CAD build for the part. Positions are in the model's coordinates, mm. Coordinates: 2 decimals unless noted, no trailing zeros. Loops run counter-clockwise (first coordinate to the right, second up) from the corner with the lowest first, then second, coordinate; pieces in that order, holes last. Notation, with made-up numbers: M -32.75,62 L -3.75,62 A7 ccw -3.75,69 Z; hole C -15.5,-17.5 d8. An arc over 180 degrees is marked long. Answer as a JSON object with one key per item and string values. Group by question number.
Autodesk Inventor part; units mm, degrees
ref_plane "YZ Plane" through (0, 0, 0) normal (1, 0, 0) x (0, 1, 0)
ref_plane "XZ Plane" through (0, 0, 0) normal (0, 1, 0) x (-1, 0, 0)
ref_plane "XY Plane" through (0, 0, 0) normal (0, 0, 1) x (1, 0, 0)
sketch "Sketch1" plane through (0, 0, 0) normal (0, 1, 0) x (-1, 0, 0)
  line L0 (50, 50) -> (-50, 50)
  line L1 (-50, 50) -> (-50, -50)
  line L2 (-50, -50) -> (50, -50)
  line L3 (50, -50) -> (50, 50)
  line L4 (50, 50) -> (-50, -50) construction
  line L5 (-50, 50) -> (50, -50) construction
  line L6 (100, 100) -> (-100, 100)
  line L7 (-100, 100) -> (-100, -100)
  line L8 (-100, -100) -> (100, -100)
  line L9 (100, -100) -> (100, 100)
  line L10 (100, 100) -> (-100, -100) construction
  line L11 (-100, 100) -> (100, -100) construction
  line L12 (-50, 100) -> (-260, 100)
  line L13 (-260, 100) -> (-260, -100)
  line L14 (-260, -100) -> (-50, -100)
  line L15 (-50, -100) -> (-50, 100)
  point P0 (0, 0)
  dimension "d0" = 100
  dimension "d1" = 100
  dimension "d2" = 200
  dimension "d3" = 50
  dimension "d4" = 210
  dimension "d5" = 0
  dimension "d6" = 200
extrude "Extrusion1" add sketch "Sketch1" along normal blind 3 contours L0 L15 L6 L9 L8 L2 L3 | L1 L15 L8 L7 L6 | L7 L14 L13 L12
sketch "Sketch3" plane through (0, 0, 0) normal (0, -1, 0) x (1, 0, 0)
  line L0 (110, 96) -> (-96, 96)
  line L1 (-96, 96) -> (-96, -96)
  line L2 (-96, -96) -> (110, -96)
  line L3 (110, -96) -> (110, 96)
  line L4 (-94, -94) -> (108, -94)
  line L5 (108, -94) -> (108, 94)
  line L6 (108, 94) -> (-94, 94)
  line L7 (-94, 94) -> (-94, -94)
  line L8 (-100, -100) -> (-100, 100)
  line L9 (260, -100) -> (-100, -100)
  line L10 (-100, 100) -> (260, 100)
  line L11 (260, 100) -> (260, -100)
  line L12 (108, 94) -> (110, 94)
  line L13 (108, -94) -> (110, -94)
  line L14 (-96, 96) -> (-81, 96)
  line L15 (-81, 96) -> (-81, 81)
  line L16 (-81, 81) -> (-96, 81)
  line L17 (-96, 81) -> (-96, 96)
  line L18 (-96, -96) -> (-81, -96)
  line L19 (-81, -96) -> (-81, -81)
  line L20 (-81, -81) -> (-96, -81)
  line L21 (-96, -81) -> (-96, -96)
  point P0 (0, 0)
  point P1 (-81, -94)
  point P2 (-94, -81)
  point P3 (-94, 81)
  point P4 (-81, 94)
  dimension "d13" = 2
  dimension "d14" = 2
  dimension "d15" = 4
  dimension "d16" = 4
  dimension "d17" = 4
  dimension "d18" = 2
  dimension "d19" = 150
  dimension "d20" = 2
  dimension "d21" = 15
  dimension "d22" = 15
  dimension "d23" = 15
  dimension "d24" = 15
extrude "Extrusion3" cut sketch "Sketch3" against normal blind 10 contours L3 L12 L6 L15 L0 | L3 L2 L19 L4 L13 | L16 L7 L20 L1
equation "\"d14\" = d13"
equation "\"d18\" = d13"
equation "\"d20\" = d14"
equation "\"d24\" = d21"
properties part number "BottomPlateRS3" material "Steel"
Item 1: Slice it at B-B, the plane z = -30. Write the cut outline in (x, y), then the cut area to 3 significant figures.
Item 2: Slice it at A-A, the plane x = 17.5. Write the cut outline in (y, z), then the cut area to 3 significant figures.
Item 3: Drill centre lines: L1, parallel to X at y = 1.25, z = 40; L2, parallel to Z at x = 42.5, y = 2.2; L3, parallel to X at y = 1.7, z = -75. Where is each one in solid material? Low to high. Write a range as from..to.
Item 4: Pin check, flat tips, straight feed: pin 1 (1 mm diameter, centred on x = 163, z = 4.5, fed in from -Y); pin 2 (12 mm diameter, centred on x = 39, z = 13.5, fed in from +Y). Stop position of each tip, or through.
Item 5: Slice it at C-C, the plane y = 1.85. Write the cut outline in (x, z), then the cut area to 3 significant figures.
Item 6: Slice it at D-D, the plane x = 54.5. Write the cut outline in (y, z), then the cut area to 3 significant figures.
Computed:
{
 "1": {"outline": "M -100,0 L -96,0 L -96,3 L -100,3 Z; M -94,0 L -50,0 L -50,3 L -94,3 Z; M 50,0 L 260,0 L 260,3 L 50,3 Z", "area": "774 mm2"},
 "2": {"outline": "M 0,-100 L 3,-100 L 3,-96 L 0,-96 Z; M 0,-94 L 3,-94 L 3,-50 L 0,-50 Z; M 0,50 L 3,50 L 3,94 L 0,94 Z; M 0,96 L 3,96 L 3,100 L 0,100 Z", "area": "288 mm2"},
 "3": {"L1": "-100..-96, -94..-50, 50..260", "L2": "-100..-96, -94..-50, 50..94, 96..100", "L3": "-100..-96, -94..260"},
 "4": {"pin 1": "y = 0", "pin 2": "through"},
 "5": {"outline": "M -100,-100 L 260,-100 L 260,100 L -100,100 Z; hole M -96,-81 L -94,-81 L -94,81 L -96,81 Z; hole M -81,-96 L 110,-96 L 110,-94 L -81,-94 Z; hole M -81,94 L 110,94 L 110,96 L -81,96 Z; hole M -50,-50 L 50,-50 L 50,50 L -50,50 Z", "area": "60,900 mm2"},
 "6": {"outline": "M 0,-100 L 3,-100 L 3,-96 L 0,-96 Z; M 0,-94 L 3,-94 L 3,94 L 0,94 Z; M 0,96 L 3,96 L 3,100 L 0,100 Z", "area": "588 mm2"}
}
